Design review of the part shown in the three views and the two pictorial views. Dimensions are in mm from the part's minimum x, y and z. Round coordinates to 2 decimals unless told otherwise and drop trailing zeros. Loops run counter-clockwise (first coordinate to the right, second up) from the corner with the lowest first, then second, coordinate; pieces in that order, holes last. Notation, with made-up numbers: M 21.5,59.5 L 40.5,59.5 A26 ccw 40.5,79.5 Z; hole C -10.75,32 d6. An arc over 180 degrees is marked long. One line per question, with ' | ' between items. Start each with the question number.
1) For probe 1 along Z at (x, y) = (50.8, 1.6); probe 2 along X at (y, z) = (2.95, 51) (1 decimal); probe 3 along X at (y, z) = (0.7, 39) (1 decimal), list the stretches that pass through material, from the lowest coordinate up. Write a range as from..to.
2) We need section B-B (z = 50.8). Give the boundary of the cut face in (x, y) (1 decimal), and give its area (3 significant figures).
3) We need section C-C (y = 2.3). Give the boundary of the cut face in (x, z) (1 decimal).
4) We need section A-A (x = 50.8). Give the boundary of the cut face in (y, z) (1 decimal).
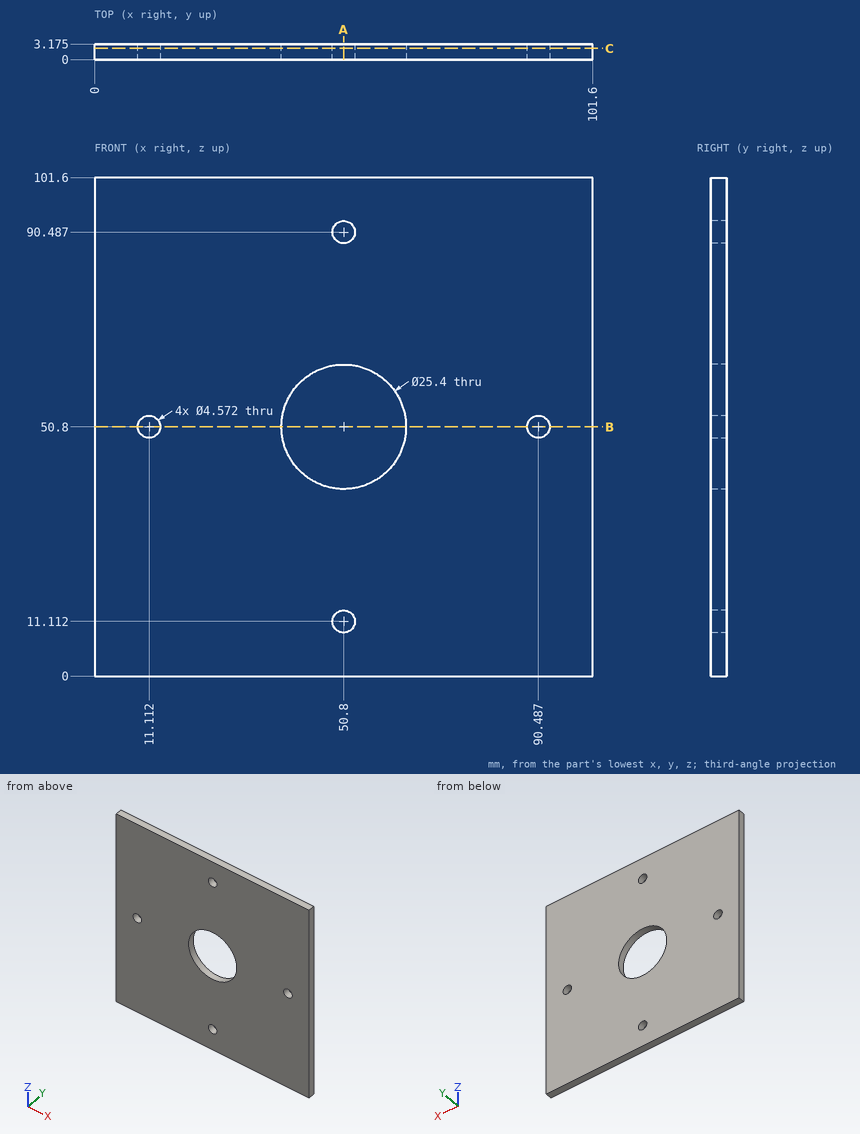
Answers below:
1) probe 1: 0..8.83, 13.4..38.1, 63.5..88.2, 92.77..101.6 | probe 2: 0..8.8, 13.4..38.1, 63.5..88.2, 92.8..101.6 | probe 3: 0..46.1, 55.5..101.6
2) outline: M 0,0 L 8.8,0 L 8.8,3.2 L 0,3.2 Z; M 13.4,0 L 38.1,0 L 38.1,3.2 L 13.4,3.2 Z; M 63.5,0 L 88.2,0 L 88.2,3.2 L 63.5,3.2 Z; M 92.8,0 L 101.6,0 L 101.6,3.2 L 92.8,3.2 Z | area: 213 mm^2
3) outline: M 0,0 L 101.6,0 L 101.6,101.6 L 0,101.6 Z; hole C 11.1,50.8 d4.6; hole C 50.8,50.8 d25.4; hole C 50.8,11.1 d4.6; hole C 50.8,90.5 d4.6; hole C 90.5,50.8 d4.6
4) outline: M 0,0 L 3.2,0 L 3.2,8.8 L 0,8.8 Z; M 0,13.4 L 3.2,13.4 L 3.2,38.1 L 0,38.1 Z; M 0,63.5 L 3.2,63.5 L 3.2,88.2 L 0,88.2 Z; M 0,92.8 L 3.2,92.8 L 3.2,101.6 L 0,101.6 Z
